Answer from the drawing. Dimensions are ordinates in mm from the lowest x, y and z of the part. A direction names the side the tool comes from. Round coordinates to 2 decimals unless told otherwise and drop trailing zeros. Order: outer loops, then holes, each group sorted by start corner. A loop starts at its lowest first (then second) coordinate and runs counter-clockwise, first axis right, second up. Notation, with made-up numbers: M 52,-35.5 L 57,-35.5 A26 ccw 57,-8.5 Z; hole C 42,27.5 d8. An arc over 180 degrees is marked long. Write item = value, one per line. Start each with the question number.
(1) A cutting plane is placed at D-D, the plane x = 23.5. Determine the outline of the cut face in (y, z).
(2) A cutting plane is placed at A-A, the plane x = 37. Determine the outline of the cut face in (y, z).
(3) A cutting plane is placed at B-B, the plane y = 1.5. Determine the outline of the cut face in (x, z), and give its area (3 significant figures).
(4) A cutting plane is placed at C-C, the plane z = 3. Determine the outline of the cut face in (x, y), and give its area (3 significant figures).
(5) Which of the six approach directions +Z, -Z, +X, -X, +Y, -Y give full straight-line access (tool end or side, diameter ignored) to the marked faces 3 and 4?
(6) Straight lines are drawn through the part: probe 1 along Z at (x, y) = (37, 1.9); probe 2 along X at (y, z) = (1.15, 3); probe 3 along Z at (x, y) = (4, 2.75). For each, find the intervals that lie inside material, in ascending order. Write a range as from..to.
(7) Each of these flat-tipped pins is pushed along its axis until it touches: pin 1 (2.5 mm diameter, centred on x = 37, z = 3, fed in from -Y); pin 2 (5 mm diameter, centred on x = 37, z = 17, fed in from +Y); pin 3 (1.5 mm diameter, centred on y = 7.5, z = 8.5, fed in from -X). Where does it stop, or does it pass through?
(8) For a pull along X with two mould halves and no side action, classify the marked faces 1 and 2 as released by +X, released by -X, zero draft, split by the parting line, or undercut.
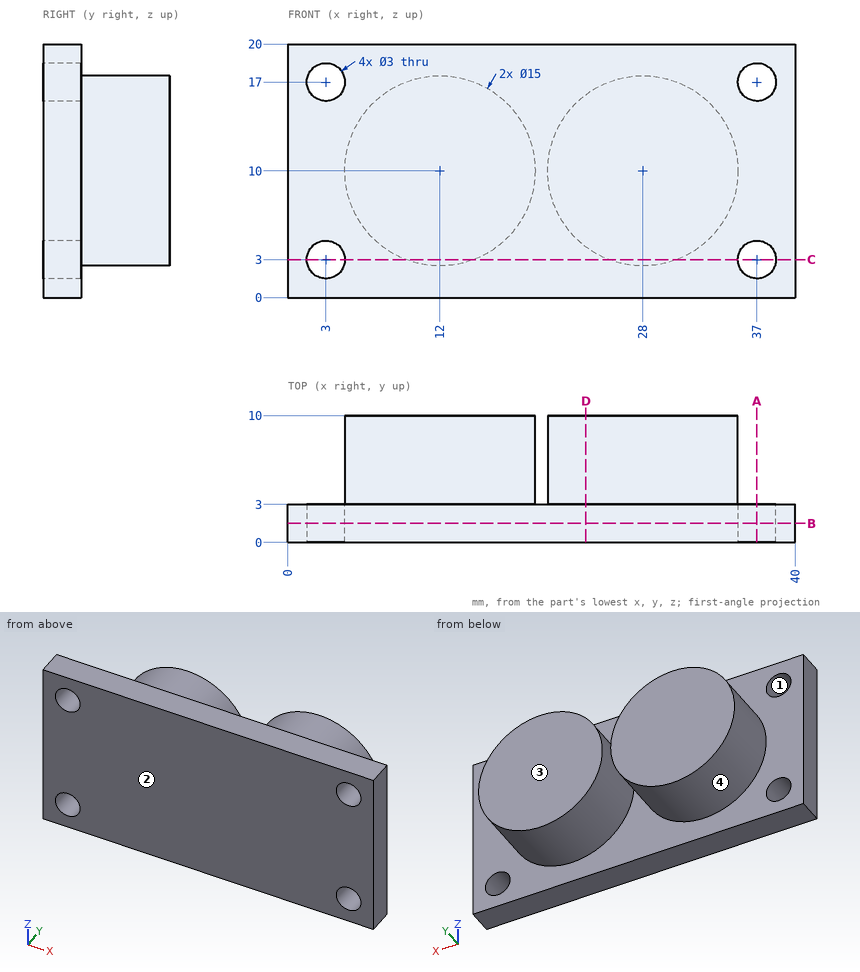
Reported:
q1.outline = M 0,0 L 3,0 L 3,4 L 10,4 L 10,16 L 3,16 L 3,20 L 0,20 Z
q2.outline = M 0,0 L 3,0 L 3,1.5 L 0,1.5 Z; M 0,4.5 L 3,4.5 L 3,15.5 L 0,15.5 Z; M 0,18.5 L 3,18.5 L 3,20 L 0,20 Z
q3.outline = M 0,0 L 40,0 L 40,20 L 0,20 Z; hole C 3,3 d3; hole C 3,17 d3; hole C 37,3 d3; hole C 37,17 d3
q3.area = 772 mm²
q4.outline = M 0,0 L 1.5,0 L 1.5,3 L 0,3 Z; M 4.5,0 L 35.5,0 L 35.5,3 L 30.69,3 L 30.69,10 L 25.31,10 L 25.31,3 L 14.69,3 L 14.69,10 L 9.31,10 L 9.31,3 L 4.5,3 Z; M 38.5,0 L 40,0 L 40,3 L 38.5,3 Z
q4.area = 177 mm²
q5.face_3 = +Z, -Z, +X, -X, +Y
q5.face_4 = +Y
q6.probe_1 = 0..1.5, 4.5..15.5, 18.5..20
q6.probe_2 = 0..1.5, 4.5..35.5, 38.5..40
q6.probe_3 = 0..1.88, 4.12..15.88, 18.12..20
q7.pin_1 = through
q7.pin_2 = 3
q7.pin_3 = 4.54
q8.face_1 = undercut
q8.face_2 = zero draft
